Study the drawing (mm; zero at the part's minimum x, y, z) and answer. Give positions to 0.01 mm unless a question says otherwise; leave off trailing zeros. Order: outer loops, then holes, each group sorted by start corner. A loop starts at its lowest first (then second) coordinate and runs counter-clockwise, first axis right, second up. Notation, with made-up numbers: (85, 33.25) - (106, 33.25) arc R20 cw to (106, 71.25) - close; hole circle Ø7 at (67.25, 51). An arc over 180 degrees is marked (long way). Return JSON: item names as keys, results as strings.
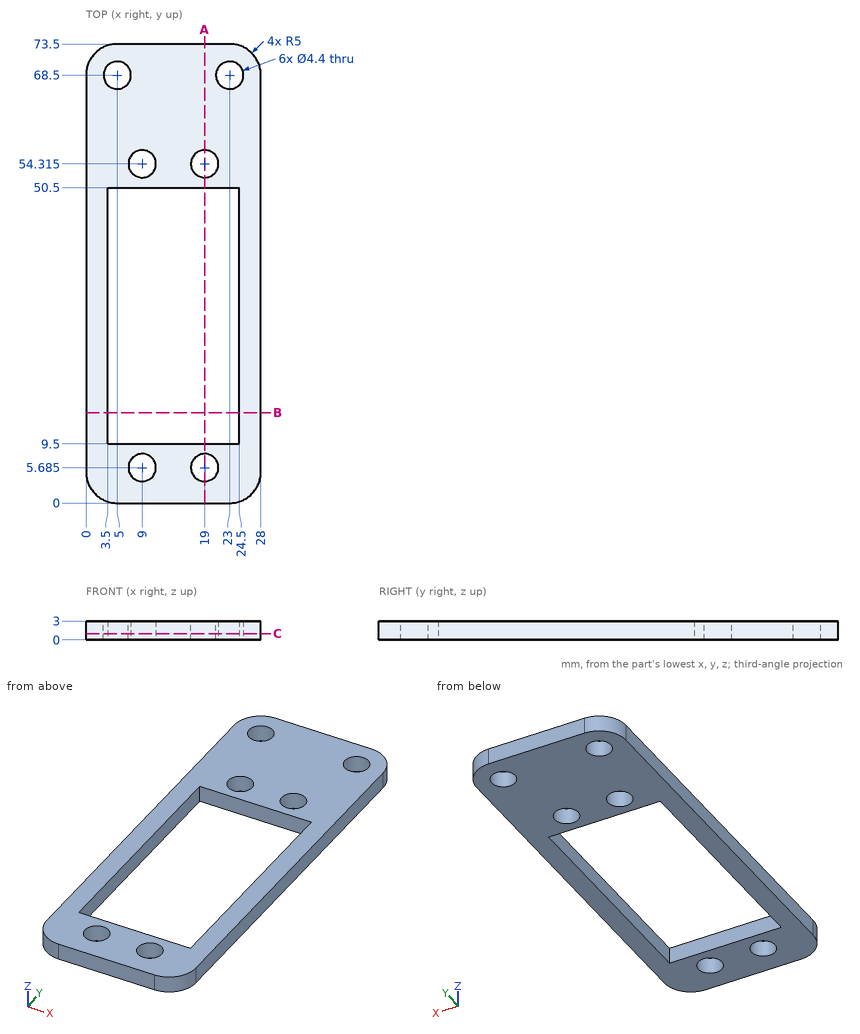
Q1. A cutting plane is placed at B-B (y = 14.5). Write down the section's boundary in (x, z).
Values:
{"outline": "(0, 0) - (3.5, 0) - (3.5, 3) - (0, 3) - close; (24.5, 0) - (28, 0) - (28, 3) - (24.5, 3) - close"}
Q2. Consider L1, parallel to Y at x = 5, z = 1.3; L2, parallel to Y at x = 19, z = 2.15 (3 decimals); L3, parallel to X at y = 25.5, z = 1.1. Determine where each line is inside the solid, lowest interval first.
Values:
{"L1": "y = 0 to 9.5, 50.5 to 66.3, 70.7 to 73.5", "L2": "y = 0 to 3.485, 7.885 to 9.5, 50.5 to 52.115, 56.515 to 73.5", "L3": "x = 0 to 3.5, 24.5 to 28"}
Q3. A cutting plane is placed at C-C (z = 1). Write down the section's boundary in (x, y) (3 decimals), and give its area (3 significant figures).
Values:
{"outline": "(0, 5) arc R5 ccw to (5, 0) - (23, 0) arc R5 ccw to (28, 5) - (28, 68.5) arc R5 ccw to (23, 73.5) - (5, 73.5) arc R5 ccw to (0, 68.5) - close; hole circle Ø4.4 at (5, 68.5); hole (3.5, 9.5) - (24.5, 9.5) - (24.5, 50.5) - (3.5, 50.5) - close; hole circle Ø4.4 at (9, 5.685); hole circle Ø4.4 at (9, 54.315); hole circle Ø4.4 at (19, 5.685); hole circle Ø4.4 at (19, 54.315); hole circle Ø4.4 at (23, 68.5)", "area": "1,080 mm²"}
Q4. Given pin 1 (4 mm diameter, centred on x = 23, y = 68.5, fed in from -Z), flat-ended and moving along its own axis, determine where the tip first touches the part or whether it passes through.
Values:
{"pin 1": "passes through"}
Q5. A cutting plane is placed at A-A (x = 19). Write down the section's boundary in (y, z) (3 decimals), and give its area (3 significant figures).
Values:
{"outline": "(0, 0) - (3.485, 0) - (3.485, 3) - (0, 3) - close; (7.885, 0) - (9.5, 0) - (9.5, 3) - (7.885, 3) - close; (50.5, 0) - (52.115, 0) - (52.115, 3) - (50.5, 3) - close; (56.515, 0) - (73.5, 0) - (73.5, 3) - (56.515, 3) - close", "area": "71.1 mm²"}
